Verification items for this drawing (mm, ordinates from the low corner). Round coordinates to 2 decimals unless told otherwise and drop trailing zeros. Order: outer loops, then holes, each group sorted by start corner. A loop starts at its lowest first (then second) coordinate and runs counter-clockwise, first axis right, second up. Notation, with made-up numbers: (-18.5, 89.25) -> (-8.5, 89.25) arc R7 cw to (-8.5, 102.25) -> close; hole circle Ø10 at (16, 19). An arc over 180 degrees is marked (long way). Use a Markdown table: item, result. Add a question column.
Item 1: Mould release check, pull along Z, two halves, no side actions. Record for the marked faces 1 and 2: pulls with the +Z half, pulls with the -Z half, needs draft (parallel to the pull), parting line crosses it, or undercut.
Item 2: Sectioned sample at A-A, the plane z = 3. Record the cut outline in (x, y).
Item 3: Material ranges on probe 1 along X at (y, z) = (118, 10.5) (1 decimal); probe 2 along X at (y, z) = (205, 4.5) (1 decimal); probe 3 along Y at (x, z) = (171.45, 7) (1 decimal), recorded low to high. Write a range as [from, to].
Item 4: Sectioned sample at B-B, the plane y = 171.45. Record the cut outline in (x, z), and give its area (3 significant figures).
Item 5: Gauge pin test, flat ends, axial feed: pin 1 Ø1 at (x, z) = (308, 10) entering from +Y; pin 2 Ø2 at (y, z) = (124.5, 4.5) entering from -X. Record the tip position at first contact, or that the pin passes through.
Item 6: Sectioned sample at D-D, the plane x = 259. Record the cut outline in (y, z).
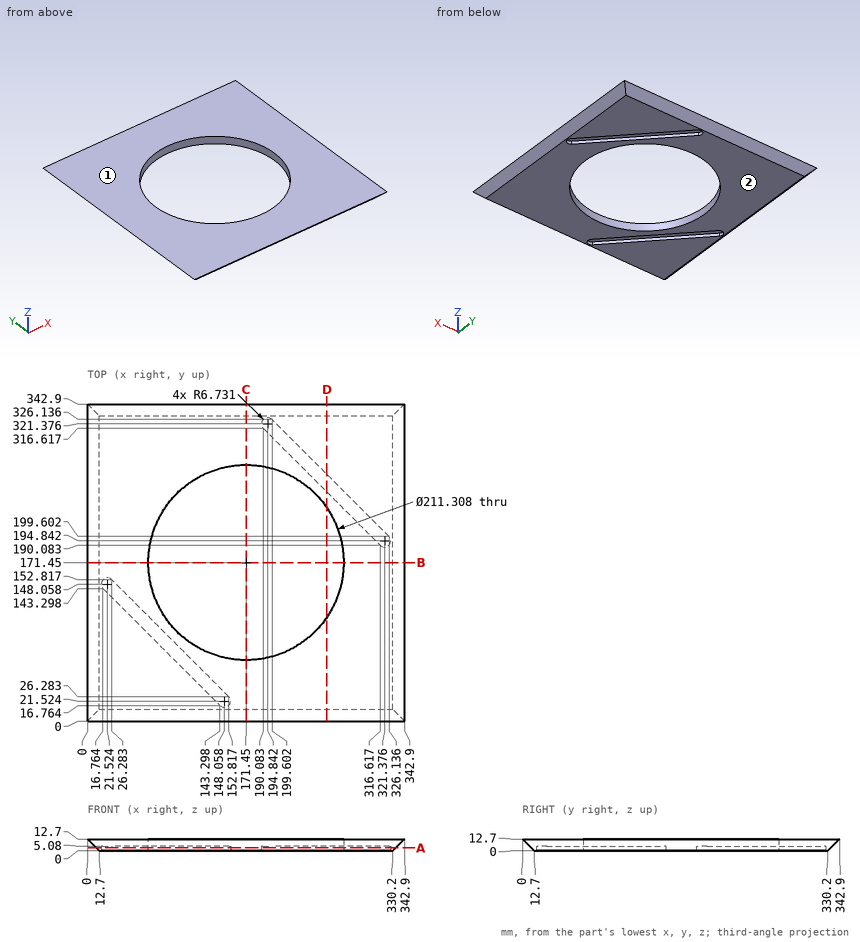
Found:
| question | item | result |
|---|---|---|
| 1 | face 1 | pulls with the +Z half |
| 1 | face 2 | pulls with the -Z half |
| 2 | outline | (9.7, 9.7) -> (333.2, 9.7) -> (333.2, 333.2) -> (9.7, 333.2) -> close; hole (16.76, 143.3) -> (143.3, 16.76) arc R6.73 ccw to (152.82, 26.28) -> (26.28, 152.82) arc R6.73 ccw to start; hole circle Ø211.31 at (171.45, 171.45); hole (190.08, 316.62) -> (316.62, 190.08) arc R6.73 ccw to (326.14, 199.6) -> (199.6, 326.14) arc R6.73 ccw to start |
| 3 | probe 1 | x = [2.2, 80.3], [262.6, 340.7] |
| 3 | probe 2 | x = [8.2, 71.3], [271.6, 301.7], [320.7, 334.7] |
| 3 | probe 3 | y = [5.7, 65.8], [277.1, 337.2] |
| 4 | outline | (0, 12.7) -> (12.7, 0) -> (65.8, 0) -> (65.8, 12.7) -> close; (277.1, 0) -> (330.2, 0) -> (342.9, 12.7) -> (277.1, 12.7) -> close |
| 4 | area | 1,510 mm2 |
| 5 | pin 1 | stops at y = 340.7 |
| 5 | pin 2 | stops at x = 7.2 |
| 6 | outline | (0, 12.7) -> (12.7, 0) -> (112.31, 0) -> (112.31, 12.7) -> close; (230.59, 0) -> (247.7, 0) -> (247.7, 5.08) -> (266.74, 5.08) -> (266.74, 0) -> (330.2, 0) -> (342.9, 12.7) -> (230.59, 12.7) -> close |
